The listing builds one solid part. Answer for the finished solid, in the listing's coordinates (mm). A direction names the side the tool comes from. Round coordinates to 2 decimals unless told otherwise and drop trailing zeros. Write each loop counter-clockwise with the first axis right and the second up, starting at its lowest first coordinate (ties: lowest second). Pieces come first, ordered by that corner, then holes.
from build123d import *

# Parameters (mm, degrees)
SKETCH_1_W          = 52.5
SKETCH_1_H          = 5.5
EXTRUDE_1_DEPTH     = 1.5
SKETCH_2_W          = 50.5
SKETCH_2_H          = 3.5
EXTRUDE_2_DEPTH     = 1
CUT_EXTRUDE_1_DEPTH = 1


with BuildPart() as part:
    # 草图1 → 凸台-拉伸1 (new body)
    with BuildSketch(Plane(origin=(0, 0, 0), x_dir=(1, 0, 0), z_dir=(0, 1, 0))):
        with Locations((26.25, -2.75)):
            Rectangle(SKETCH_1_W, SKETCH_1_H)
    extrude(amount=EXTRUDE_1_DEPTH)

    # 草图2 → 凸台-拉伸2 (add)
    with BuildSketch(Plane(origin=(0, 1.5, 0), x_dir=(1, 0, 0), z_dir=(0, 1, 0))):
        with Locations((26.25, -2.75)):
            Rectangle(SKETCH_2_W, SKETCH_2_H)
    extrude(amount=EXTRUDE_2_DEPTH)

    # 草图3 → 切除-拉伸1 (cut)
    with BuildSketch(Plane(origin=(0, 2.5, 0), x_dir=(1, 0, 0), z_dir=(0, 1, 0))):
        Polygon((2.441285036, -1), (2.441285036, -3.385807874), (3.297792845, -3.385807874), (3.297792845, -2.590222366), (5.010808462, -2.590222366), (5.010808462, -4.02818873), (5.797531803, -4.02818873), (5.797531803, -3.110546333), (8.253302308, -3.110546333), (8.253302308, -2.590222366), (5.813610605, -2.590222366), (5.813610605, -1.721967074), (11.771102235, -1.721967074), (11.771102235, -3.385807874), (12.90419018, -3.385807874), (12.90419018, -1), align=None)
        Polygon((13.734934002, -4.5), (13.734934002, -3.806276904), (18.57720237, -3.806276904), (18.57720237, -3.191075541), (21.800907432, -3.191075541), (21.800907432, -3.942903937), (20.000873813, -3.942903937), (20.000873813, -4.5), align=None)
        Polygon((16.237613485, -1), (16.237613485, -1.73768688), (22.365277211, -1.73768688), (22.365277211, -3.5), (23.277541754, -3.5), (23.277541754, -1), align=None)
        Polygon((25.11928338, -1.598265318), (25.11928338, -2.796313913), (26.916272405, -2.796313913), (26.916272405, -4.02818873), (27.721819209, -4.02818873), (27.721819209, -2.371232168), (33.367210511, -2.371232168), (33.367210511, -2.796313913), (31.81151837, -2.796313913), (31.81151837, -3.519184621), (34.558639523, -3.519184621), (34.558639523, -1.598265318), (30.055839437, -1.598265318), (30.055839437, -1), (27.143477914, -1), (27.143477914, -1.598265318), align=None)
        Polygon((36.247190267, -1), (36.247190267, -2.51018455), (35.430902313, -2.51018455), (35.430902313, -3.110546333), (37.734000469, -3.110546333), (37.734000469, -1.755092275), (39.075044965, -1.755092275), (39.075044965, -3.519184621), (40.007945484, -3.519184621), (40.007945484, -1.42807574), (40.007945484, -1), align=None)
        Polygon((41.31314972, -4.5), (41.31314972, -3.749200991), (42.825396523, -3.749200991), (42.825396523, -1.755092275), (43.353482708, -1.755092275), (43.353482708, -3.519184621), (44.913737346, -3.519184621), (44.913737346, -2.873049456), (48.730360229, -2.873049456), (48.730360229, -3.5), (46.305964561, -3.5), (46.305964561, -4.185040027), (42.825396523, -4.185040027), (42.825396523, -4.5), align=None)
        Polygon((47.464486029, -1), (47.464486029, -2.039438327), (49.049976505, -2.039438327), (49.049976505, -1.42807574), (51.5, -1.42807574), (51.5, -1), align=None)
    extrude(amount=-CUT_EXTRUDE_1_DEPTH, mode=Mode.SUBTRACT)


solid = part.part
1. Section B-B on z = 4.95 is taken. Determine the outline of the cut face in (x, y).
Geometry says:
outline: (0, 0) - (52.5, 0) - (52.5, 1.5) - (0, 1.5) - close
2. Section A-A on x = 48 is taken. Determine the outline of the cut face in (y, z).
Geometry says:
outline: (0, 0) - (1.5, 0) - (1.5, 2.04) - (2.5, 2.04) - (2.5, 2.87) - (1.5, 2.87) - (1.5, 3.5) - (2.5, 3.5) - (2.5, 4.5) - (1.5, 4.5) - (1.5, 5.5) - (0, 5.5) - close
3. Section C-C on x = 7 is taken. Determine the outline of the cut face in (y, z).
Geometry says:
outline: (0, 0) - (1.5, 0) - (1.5, 1.72) - (2.5, 1.72) - (2.5, 2.59) - (1.5, 2.59) - (1.5, 3.11) - (2.5, 3.11) - (2.5, 4.5) - (1.5, 4.5) - (1.5, 5.5) - (0, 5.5) - close
4. A tool of negligible diameter and unlimited length cuts with its end or side. For faces 1 (the face through (26, 2.5, 3)), 2 (the face through (3, 2, 3.386)), 3 (the face through (34.559, 2, 3)), from which of +Z, -Z, +X, -X, +Y, -Y can it reach the whole face along a straight path? Write none if from no direction.
Geometry says:
face 1: +Z, -Z, +X, -X, +Y
face 2: -Z, +Y
face 3: +Y
5. For a pull along X with two mould halves and no side action, classify faces 4 (the face through (0, 1, 3)), 5 (the face through (44, 2, 3.519)), 6 (the face through (51.5, 2, 3)), 7 (the face through (2, 2, 1)) as released by +X, released by -X, zero draft, split by the parting line, or undercut.
Geometry says:
face 4: released by -X
face 5: undercut
face 6: released by +X
face 7: zero draft
6. Straight lines are drawn through the part: line 1 along X through (y, z) = (1.9, 3.55); line 2 along Z through (x, y) = (45, 1.65); line 3 along Y through (x, z) = (15.5, 0.7). For each, find the intervals that lie inside material, in ascending order.
Geometry says:
line 1: x = 1 to 5.01, 5.8 to 18.58, 21.8 to 26.92, 27.72 to 42.83, 46.31 to 51.5
line 2: z = 1 to 2.87, 4.19 to 4.5
line 3: y = 0 to 1.5
7. Given pin 1 (0.5 mm diameter, centred on x = 42.5, y = 2, fed in from -Z); pin 2 (0.8 mm diameter, centred on y = 2, z = 2.5, fed in from -X); pin 3 (0.5 mm diameter, centred on x = 33, y = 2, fed in from +Z), each flat-ended and moving along its own axis, determine where each tip first touches the part or whether it passes through.
Geometry says:
pin 1: stops at z = 1
pin 2: stops at x = 1
pin 3: stops at z = 4.5
